Input: dimensioned drawing with shaded views. Units: mm. Origin: part minimum x, y, z. A direction names the side the tool comes from. Round coordinates to 2 decimals unless told otherwise and drop trailing zeros. Order: outer loops, then holes, each group sorted by start corner. A loop starts at its lowest first (then second) coordinate and runs counter-clockwise, first axis right, second up. Notation, with made-up numbers: (43, -9.5) - (56, -9.5) arc R21 cw to (56, 10.5) - close; hole circle Ø2 at (22.25, -26). An arc over 180 degrees is marked (long way). Return JSON: item names as keys, results as strings. Group by question number.
1) Section C-C, the plane y = 10. Return loops of the section in (x, z), plus the area to 3 significant figures.
2) Section A-A, the plane z = 16. Return loops of the section in (x, y), plus the area to 3 significant figures.
3) Ray query, line 1 (Y direction, x = 14, z = 6.75); line 2 (Y direction, x = 30.1, z = 3.9); line 3 (Z direction, x = 0.85, y = 10). Return the intervals inside material, ascending. Write a range as from..to.
4) Contact query for flat-ended pins moving along their axis: P1, Ø6, axis at x = 9, y = 10.5, coming from the +Z side; P2, Ø5.5, axis at y = 11, z = 7.5, coming from the +X side; P3, Ø2.5, axis at x = 15, z = 6.5, coming from the +Y side; P4, Ø6, axis at y = 9.5, z = 15, coming from the +X side. Output: stop coordinate, or through.
5) Section D-D, the plane x = 14. Return loops of the section in (y, z).
6) Section B-B, the plane x = 30.1. Return loops of the section in (y, z).
7) Access query for the marked faces 1, 2 and 3. Directions: +Z, -Z, +X, -X, +Y, -Y. A direction counts if a zero-diameter tool reaches every point of the face in a straight line with its end or side. Return the directions, or none.
8) Mould query, pull axis Y, two halves, no side actions, for the marked faces 4, 5, 6 and 7. Classes: pulls with the +Y half, pulls with the -Y half, needs draft (parallel to the pull), parting line crosses it, or undercut.
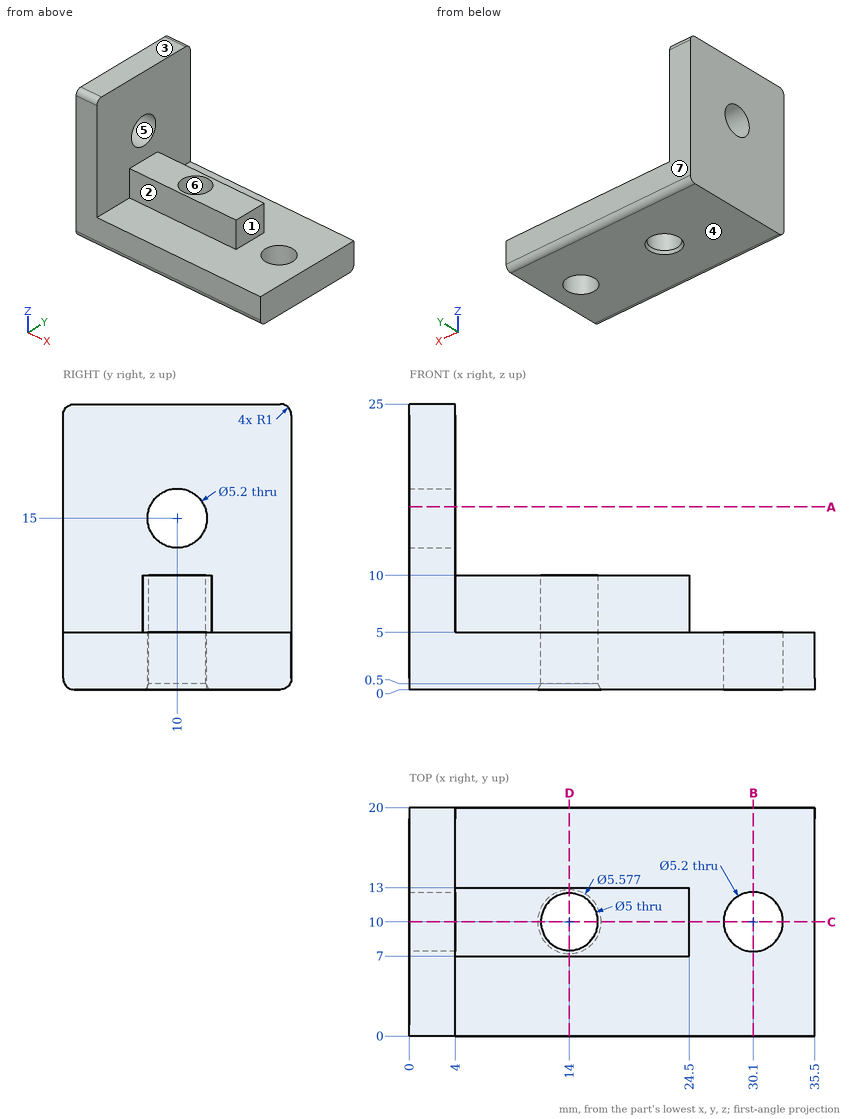
Geometry check:
{
 "1": {"outline": "(0, 0) - (11.21, 0) - (11.5, 0.5) - (11.5, 10) - (4, 10) - (4, 12.4) - (0, 12.4) - close; (0, 17.6) - (4, 17.6) - (4, 25) - (0, 25) - close; (16.5, 0.5) - (16.79, 0) - (27.5, 0) - (27.5, 5) - (24.5, 5) - (24.5, 10) - (16.5, 10) - close; (32.7, 0) - (35.5, 0) - (35.5, 5) - (32.7, 5) - close", "area": "263 mm2"},
 "2": {"outline": "(0, 0) - (4, 0) - (4, 7.6) - (0, 7.6) - close; (0, 12.4) - (4, 12.4) - (4, 20) - (0, 20) - close", "area": "60.8 mm2"},
 "3": {"line 1": "7..7.5, 12.5..13", "line 2": "0..7.4, 12.6..20", "line 3": "0..12.4, 17.6..25"},
 "4": {"P1": "z = 10", "P2": "x = 35.5", "P3": "y = 13", "P4": "x = 4"},
 "5": {"outline": "(0, 1) arc R1 ccw to (1, 0) - (7.21, 0) - (7.5, 0.5) - (7.5, 10) - (7, 10) - (7, 5) - (0, 5) - close; (12.5, 0.5) - (12.79, 0) - (19, 0) arc R1 ccw to (20, 1) - (20, 5) - (13, 5) - (13, 10) - (12.5, 10) - close"},
 "6": {"outline": "(0, 1) arc R1 ccw to (1, 0) - (7.4, 0) - (7.4, 5) - (0, 5) - close; (12.6, 0) - (19, 0) arc R1 ccw to (20, 1) - (20, 5) - (12.6, 5) - close"},
 "7": {"face 1": "+Z, +X, +Y, -Y", "face 2": "+Z, +X, -Y", "face 3": "+Z, +X, -X, +Y, -Y"},
 "8": {"face 4": "needs draft", "face 5": "undercut", "face 6": "undercut", "face 7": "pulls with the +Y half"}
}
